from build123d import *

# Parameters (mm, degrees)
BOSS_EXTRUDE1_DEPTH        = 3.175
F_9_0_196_DIAMETER_HOLE1_D = 4.9784


with BuildPart() as part:
    # Sketch1 → Boss-Extrude1 (new body)
    with BuildSketch(Plane(origin=(0, 0, 0), x_dir=(0, 1, 0), z_dir=(0, 0, 1))):
        with BuildLine():
            Line((-12.7, -49.151299627), (-12.7, 40.764697174))
            ThreePointArc((-12.7, 40.764697174), (0, 53.464697174), (12.7, 40.764697174))
            Line((12.7, 40.764697174), (12.7, -49.151302826))
            ThreePointArc((12.7, -49.151302826), (-1.599e-06, -61.851302826), (-12.7, -49.151299627))
        make_face()
    extrude(amount=BOSS_EXTRUDE1_DEPTH)

    # #9 (0.196) Diameter Hole1 (through all)
    with Locations(Plane.XY.offset(3.175)):
        with Locations((-40.764697174, 0), (49.151302826, 0)):
            Hole(F_9_0_196_DIAMETER_HOLE1_D / 2)


solid = part.part
CAD build for the part. Positions are in the model's coordinates, mm. Round coordinates to 2 decimals unless told otherwise and drop trailing zeros. Loops run counter-clockwise (first coordinate to the right, second up) from the corner with the lowest first, then second, coordinate; pieces in that order, holes last.
(1) Cut at A-A (z = 1.95). Give the cut face in (x, y), plus the area to 3 significant figures.
(2) Cut at B-B (y = 0). Give the cut face in (x, z) (1 decimal).
(3) Two-plate mould, pull along Y, no slides. Class faces 1 (the cylindrical face through (51.64, 0.11, 1.57)), 2 (the cylindrical face through (-43.064, -0.953, 1.565)), 3 (the cylindrical face through (-53.46, -0.28, 1.57)), 4 (the flat face through (3, 0, 3.175)): +Y half, -Y half, draft (parallel to the pull), parting line (faces both ways), or undercut.
(4) Wall check: line 1 along X through (y, z) = (-0.75, 1.6); line 2 along X through (y, z) = (-1.5, 0.45); line 3 along Y through (x, z) = (47.5, 2.9). Give the ranges that are in metal, low to high.
(5) Drop a flat-ended pin along its axis: pin 1 (1 mm diameter, centred on y = 1.5, z = 2, fed in from -X). Give the stop position or say it passes through.
(6) Cut at C-C (y = 8.5). Give the cut face in (x, z) (3 decimals), plus the area to 3 significant figures.
Findings below:
1. outline: (-40.76, -12.7) - (49.15, -12.7) arc R12.7 ccw to (49.15, 12.7) - (-40.76, 12.7) arc R12.7 ccw to start; hole circle Ø4.98 at (-40.76, 0); hole circle Ø4.98 at (49.15, 0)
1. area: 2,750 mm2
2. outline: (-53.5, 0) - (-43.3, 0) - (-43.3, 3.2) - (-53.5, 3.2) - close; (-38.3, 0) - (46.7, 0) - (46.7, 3.2) - (-38.3, 3.2) - close; (51.6, 0) - (61.9, 0) - (61.9, 3.2) - (51.6, 3.2) - close
3. face 1: undercut
3. face 2: undercut
3. face 3: parting line
3. face 4: draft
4. line 1: x = -53.44 to -43.14, -38.39 to 46.78, 51.52 to 61.83
4. line 2: x = -53.38 to -42.75, -38.78 to 47.16, 51.14 to 61.76
4. line 3: y = -12.7 to -1.86, 1.86 to 12.7
5. pin 1: stops at x = -53.43
6. outline: (-50.201, 0) - (58.587, 0) - (58.587, 3.175) - (-50.201, 3.175) - close
6. area: 345 mm2
